Here's how the part is built. I have some questions about the finished solid (model axes, mm). Face numbers are marked on the shaded views. A direction names the side the tool comes from. Round coordinates to 2 decimals unless told otherwise and drop trailing zeros. Order: outer loops, then holes, each group sorted by start corner. A loop starts at its lowest first (then second) coordinate and runs counter-clockwise, first axis right, second up. Notation, with made-up numbers: (29, -32) -> (47, -32) arc R26 cw to (47, 3) -> close; hole circle Ø8 at (-36, 53.25). An arc over 180 degrees is marked (long way). Use a Markdown table: item, result. Add a question column.
from build123d import *

# Parameters (mm, degrees)
F1_DEPTH  = 6.35
F0_W      = 11.43
F0_H      = 7.62
F0_W_2    = 7.62
F2_DEPTH  = 19.05
F3_DEPTH  = 19.05
F4_DEPTH  = 12.7
F6_DEPTH  = 127
F8_D      = 18.542
F8_DEPTH  = 7.62
F8_TIP    = 5.570578799
F10_D     = 14.8336
F10_DEPTH = 7.62
F10_TIP   = 4.4564630392
F11_W     = 8.128
F11_H     = 1.778
F11_H_2   = 3.556
F11_H_3   = 3.81
F12_DEPTH = 3.556
F9_W      = 12.7
F9_H      = 7.62
F15_DEPTH = 76.201
F13_R     = 1.5875
F14_R     = 1.5875
F16_DEPTH = 38.1
F18_R     = 1.5875
F20_R     = 1.5875
F19_R     = 1.5875
F21_DEPTH = 2.794
F22_DEPTH = 2.794


# Not quite as in the source:
# - a feature names something its author has since deleted; it is built from what else it names


with BuildPart() as f1:
    # F0 (on Front) → F1 (new body, symmetric)
    with BuildSketch(Plane.XZ):
        Polygon((49.53, 38.1), (-49.53, 38.1), (-37.6766666667, 30.48), (37.6766666667, 30.48), align=None)
        Polygon((-37.6766666667, -30.48), (-49.53, -38.1), (49.53, -38.1), (37.6766666667, -30.48), align=None)
        Polygon((-49.53, 25.5814285714), (-57.15, 30.48), (-57.15, -30.48), (-49.53, -25.5814285714), align=None)
        Polygon((-49.53, 30.48), (-57.15, 30.48), (-49.53, 25.5814285714), align=None)
        Polygon((-37.6766666667, 30.48), (-49.53, 38.1), (-49.53, 30.48), align=None)
        Polygon((49.53, 30.48), (49.53, 38.1), (37.6766666667, 30.48), align=None)
        Polygon((37.6766666667, -30.48), (49.53, -38.1), (49.53, -30.48), align=None)
        Polygon((-37.6766666667, -30.48), (-49.53, -30.48), (-49.53, -38.1), align=None)
        Polygon((-49.53, -25.5814285714), (-57.15, -30.48), (-49.53, -30.48), align=None)
        Polygon((57.15, -30.48), (57.15, 30.48), (49.53, 25.5814285714), (49.53, -25.5814285714), align=None)
        Polygon((49.53, -30.48), (57.15, -30.48), (49.53, -25.5814285714), align=None)
        Polygon((57.15, 30.48), (49.53, 30.48), (49.53, 25.5814285714), align=None)
        Polygon((49.53, 25.5814285714), (49.53, 30.48), (37.6766666667, 30.48), (0, 6.2592857143), (9.7366666667, 0), align=None)
        Polygon((49.53, -25.5814285714), (9.7366666667, 0), (0, -6.2592857143), (37.6766666667, -30.48), (49.53, -30.48), align=None)
        Polygon((-49.53, -25.5814285714), (-49.53, -30.48), (-37.6766666667, -30.48), (0, -6.2592857143), (-9.7366666667, 0), align=None)
        Polygon((-37.6766666667, 30.48), (-49.53, 30.48), (-49.53, 25.5814285714), (-9.7366666667, 0), (0, 6.2592857143), align=None)
        Polygon((9.7366666667, 0), (0, 6.2592857143), (-9.7366666667, 0), (0, -6.2592857143), align=None)
    extrude(amount=F1_DEPTH, both=True)

    # F0 (on Front) → F2 (join, symmetric)
    with BuildSketch(Plane.XZ):
        with Locations((-62.865, -34.29)):
            Rectangle(F0_W, F0_H)
        with Locations((-62.865, 34.29)):
            Rectangle(F0_W, F0_H)
        with Locations((-53.34, -34.29)):
            Rectangle(F0_W_2, F0_H)
        with Locations((-53.34, 34.29)):
            Rectangle(F0_W_2, F0_H)
    extrude(amount=F2_DEPTH, both=True)

    # F0 (on Front) → F3 (join, symmetric)
    with BuildSketch(Plane.XZ):
        Polygon((57.15, 63.5), (57.15, 38.1), (57.15, 30.48), (57.15, -30.48), (57.15, -38.1), (64.77, -38.1), (64.77, 63.5), align=None)
    extrude(amount=F3_DEPTH, both=True)

    # F0 (on Front) → F4 (join, symmetric)
    with BuildSketch(Plane.XZ):
        with Locations((53.34, 34.29)):
            Rectangle(F0_W_2, F0_H)
        with Locations((53.34, -34.29)):
            Rectangle(F0_W_2, F0_H)
    extrude(amount=F4_DEPTH, both=True)

    # F5 (on face) → F6 (cut)
    with BuildSketch(Plane.XY.offset(63.5)):
        Polygon((57.15, 14.6505909488), (64.77, 19.05), (57.15, 19.05), align=None)
        Polygon((57.15, -19.05), (64.77, -19.05), (57.15, -14.6505909488), align=None)
    extrude(amount=-F6_DEPTH, mode=Mode.SUBTRACT)

    # F8
    with Locations(Plane(origin=(0, 0, -38.1), x_dir=(1, 0, 0), z_dir=(0, 0, -1))):
        with Locations((-69.85, 0)):
            Hole(F8_D / 2, depth=F8_DEPTH)
            with Locations((0, 0, -(F8_DEPTH + F8_TIP / 2))):  # 118° drill point
                Cone(0, F8_D / 2, F8_TIP, mode=Mode.SUBTRACT)

    # F10
    with Locations(Plane.XY.offset(38.1)):
        with Locations((-69.85, 0)):
            Hole(F10_D / 2, depth=F10_DEPTH)
            with Locations((0, 0, -(F10_DEPTH + F10_TIP / 2))):  # 118° drill point
                Cone(0, F10_D / 2, F10_TIP, mode=Mode.SUBTRACT)

    # F11 (on face) → F12 (cut)
    with BuildSketch(Plane.YZ.offset(64.77)):
        with Locations((0, 62.611)):
            Rectangle(F11_W, F11_H)
        with Locations((0, 56.388)):
            Rectangle(F11_W, F11_H_2)
        with Locations((0, 49.276)):
            Rectangle(F11_W, F11_H_2)
        with Locations((0, 42.164)):
            Rectangle(F11_W, F11_H_2)
        with Locations((0, 35.052)):
            Rectangle(F11_W, F11_H_2)
        with Locations((0, 27.94)):
            Rectangle(F11_W, F11_H_2)
        with Locations((0, 20.828)):
            Rectangle(F11_W, F11_H_2)
        with Locations((0, 13.716)):
            Rectangle(F11_W, F11_H_2)
        with Locations((0, 6.604)):
            Rectangle(F11_W, F11_H_2)
        with Locations((0, -0.508)):
            Rectangle(F11_W, F11_H_2)
        with Locations((0, -7.62)):
            Rectangle(F11_W, F11_H_2)
        with Locations((0, -14.732)):
            Rectangle(F11_W, F11_H_2)
        with Locations((0, -21.844)):
            Rectangle(F11_W, F11_H_2)
        with Locations((0, -28.956)):
            Rectangle(F11_W, F11_H_2)
        with Locations((0, -36.195)):
            Rectangle(F11_W, F11_H_3)
    extrude(amount=-F12_DEPTH, mode=Mode.SUBTRACT)

    # F9 (on face) → F15 (cut, through all)
    with BuildSketch(Plane.XY.offset(38.1)):
        with Locations((-55.88, 15.24)):
            Rectangle(F9_W, F9_H)
        with Locations((-55.88, -15.24)):
            Rectangle(F9_W, F9_H)
    extrude(amount=-F15_DEPTH, mode=Mode.SUBTRACT)

    # F13 (on face) + F14 (on face) → F16 (cut)
    with BuildSketch(Plane(origin=(-68.58, 0, 0), x_dir=(0, -1, 0), z_dir=(-1, 0, 0))):
        with Locations((-15.24, 34.29)):
            Circle(F13_R)
        with Locations((15.24, 34.29)):
            Circle(F13_R)
    with BuildSketch(Plane(origin=(-68.58, 0, 0), x_dir=(0, -1, 0), z_dir=(-1, 0, 0))):
        with Locations((15.24, -34.29)):
            Circle(F14_R)
        with Locations((-15.24, -34.29)):
            Circle(F14_R)
    extrude(amount=-F16_DEPTH, mode=Mode.SUBTRACT)

    # F17 (on face) + F18 (on face) + F20 (on face) + F19 (on face) → F21 (cut)
    with BuildSketch(Plane.YZ.offset(-62.23)):
        Polygon((19.0528211777, 34.29), (17.1464105889, 37.592), (13.3335894111, 37.592), (11.4271788223, 34.29), (13.3335894111, 30.988), (17.1464105889, 30.988), align=None)
    with BuildSketch(Plane.YZ.offset(-62.23)):
        Polygon((-11.43, 34.2948864232), (-13.3335894111, 37.592), (-17.1464105889, 37.592), (-19.05, 34.2948864232), (-19.05, 34.2851135768), (-17.1464105889, 30.988), (-13.3335894111, 30.988), (-11.43, 34.2851135768), align=None)
        with Locations((-15.24, 34.29)):
            Circle(F18_R, mode=Mode.SUBTRACT)
    with BuildSketch(Plane.YZ.offset(-62.23)):
        Polygon((-11.43, -34.2851135768), (-13.3335894111, -30.988), (-17.1464105889, -30.988), (-19.05, -34.2851135768), (-19.05, -34.2948864232), (-17.1464105889, -37.592), (-13.3335894111, -37.592), (-11.43, -34.2948864232), align=None)
        with Locations((-15.24, -34.29)):
            Circle(F20_R, mode=Mode.SUBTRACT)
    with BuildSketch(Plane.YZ.offset(-62.23)):
        Polygon((19.05, -34.2851135768), (17.1464105889, -30.988), (13.3335894111, -30.988), (11.43, -34.2851135768), (11.43, -34.2948864232), (13.3335894111, -37.592), (17.1464105889, -37.592), (19.05, -34.2948864232), align=None)
        with Locations((15.24, -34.29)):
            Circle(F19_R, mode=Mode.SUBTRACT)
    extrude(amount=-F21_DEPTH, mode=Mode.SUBTRACT)

    # F18 (on face) → F22 (cut)
    with BuildSketch(Plane.YZ.offset(-62.23)):
        Polygon((-11.4271788223, 34.29), (-13.3335894111, 37.592), (-17.1464105889, 37.592), (-19.0528211777, 34.29), (-17.1464105889, 30.988), (-13.3335894111, 30.988), align=None)
    extrude(amount=-F22_DEPTH, mode=Mode.SUBTRACT)


solid = f1.part
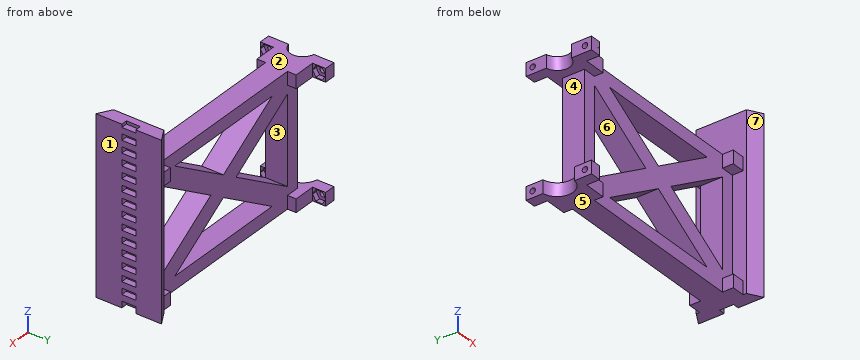
(1) Please list where these lines run through material, in increasing order: probe 1 along Z at (x, y) = (-67.65, 15.24); probe 2 along Y at (x, z) = (-67, -34); probe 3 along Y at (x, z) = (-67, 34). Write a range as from..to.
(2) On a 3-axis mill with a long thin cutter (end or side, diameter ignored), from which of +Z, -Z, +X, -X, +Y, -Y can I reach the whole of each face in a straight line? I mean the marked faces 4, 5, 6 and 7. Say none if no direction works.
(3) I want a section at A-A on x = 13.5. List the corners of the cut face in (y, z) for me, and give its area (3 significant figures).
(4) I want a section at B-B on z = 49. List the corners of the cut face in (x, y) for me, and give its area (3 significant figures).
(5) If we mould it in two halves opening along Z, with no side actions, what happens to the marked faces 1, 2 and 3? For each: pulls with the +Z half, pulls with the -Z half, needs draft (parallel to the pull), parting line crosses it, or undercut.
(6) I want a section at D-D on y = 2. State how many separate pieces and enclosed holes the cut face has, and give its area (3 significant figures).
(7) I want a section at C-C on z = -15. List the corners of the cut face in (x, y) for me.
(8) I'm going to push flat-ended pins straight in: P1, Ø4, axis at x = -13.5, z = 35.5, coming from the -Y side; P2, Ø1.1, axis at x = 63.5, y = -0.5, coming from the -Z side; P3, Ø12, axis at x = -47.5, y = -13, coming from the +Z side. Where does each tip first touch, or does it pass through?
Output:
| question | item | result |
|---|---|---|
| 1 | probe 1 | -38.1..-35.88, -32.7..-30.48, 30.48..32.7, 35.88..38.1 |
| 1 | probe 2 | -19.05..-16.8, -13.68..-8.82, 8.82..13.68, 16.8..19.05 |
| 1 | probe 3 | -19.05..-16.8, -13.68..-6.85, 6.85..13.68, 16.8..19.05 |
| 2 | face 4 | -X, +Y, -Y |
| 2 | face 5 | -Z, +X, -X, +Y, -Y |
| 2 | face 6 | +Y, -Y |
| 2 | face 7 | +Z, -Z, -Y |
| 3 | outline | (-6.35, -38.1) -> (6.35, -38.1) -> (6.35, -30.48) -> (-6.35, -30.48) -> close; (-6.35, -14.94) -> (6.35, -14.94) -> (6.35, -2.42) -> (-6.35, -2.42) -> close; (-6.35, 2.42) -> (6.35, 2.42) -> (6.35, 14.94) -> (-6.35, 14.94) -> close; (-6.35, 30.48) -> (6.35, 30.48) -> (6.35, 38.1) -> (-6.35, 38.1) -> close |
| 3 | area | 512 mm² |
| 4 | outline | (57.15, -14.65) -> (64.77, -19.05) -> (64.77, -4.06) -> (61.21, -4.06) -> (61.21, 4.06) -> (64.77, 4.06) -> (64.77, 19.05) -> (57.15, 14.65) -> close |
| 4 | area | 228 mm² |
| 5 | face 1 | needs draft |
| 5 | face 2 | pulls with the +Z half |
| 5 | face 3 | undercut |
| 6 | separate pieces | 1 |
| 6 | enclosed holes | 4 |
| 6 | area | 5,510 mm² |
| 7 | outline | (-57.15, -6.35) -> (-49.53, -6.35) -> (-49.53, 6.35) -> (-57.15, 6.35) -> close; (-33.07, -6.35) -> (-13.6, -6.35) -> (-13.6, 6.35) -> (-33.07, 6.35) -> close; (13.6, -6.35) -> (33.07, -6.35) -> (33.07, 6.35) -> (13.6, 6.35) -> close; (49.53, -6.35) -> (57.15, -6.35) -> (57.15, -14.65) -> (64.77, -19.05) -> (64.77, -4.06) -> (61.21, -4.06) -> (61.21, 4.06) -> (64.77, 4.06) -> (64.77, 19.05) -> (57.15, 14.65) -> (57.15, 6.35) -> (49.53, 6.35) -> close |
| 8 | P1 | y = -6.35 |
| 8 | P2 | z = -34.29 |
| 8 | P3 | z = 38.1 |
